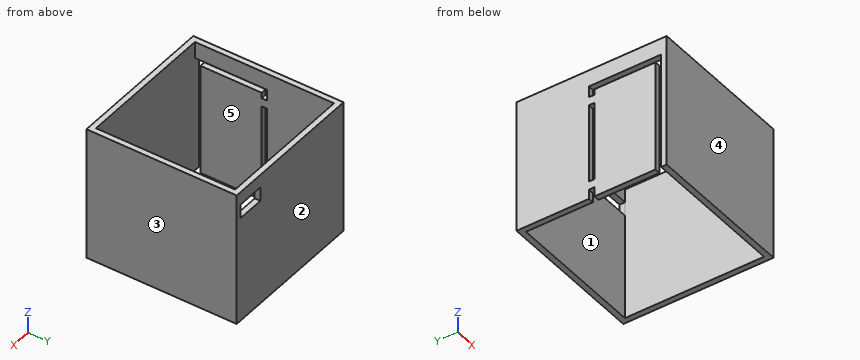
```python
from build123d import *

# Parameters (mm, degrees)
F0_W     = 50
F0_H     = 2
F1_DEPTH = 48
F3_W     = 2
F3_H     = 40
F3_H_2   = 3.4556204919
F3_H_3   = 28.4943341073
F3_H_4   = 2.0500454009
F4_DEPTH = 25
F5_W     = 10
F5_H     = 5
F6_DEPTH = 2


with BuildPart() as f1:
    # F0 (on Top) → F1 (new body)
    with BuildSketch(Plane.XY):
        with Locations((-0.1711930672, -2.4346486163)):
            Rectangle(F0_W, F0_H)
        Polygon((-27.1711930672, -3.4346486163), (-25.1711930672, -3.4346486163), (-25.1711930672, -1.4346486163), (-25.1711930672, 48.5653513837), (-25.1711930672, 50.5653513837), (-27.1711930672, 50.5653513837), align=None)
        Polygon((24.8288069328, -1.4346486163), (24.8288069328, -3.4346486163), (26.8288069328, -3.4346486163), (26.8288069328, 50.5653513837), (24.8288069328, 50.5653513837), (24.8288069328, 48.5653513837), align=None)
        with Locations((-0.1711930672, 49.5653513837)):
            Rectangle(F0_W, F0_H)
    extrude(amount=F1_DEPTH)

    # F3 (on face) → F4 (cut)
    with BuildSketch(Plane(origin=(-27.1711930672, 0, 0), x_dir=(0, -1, 0), z_dir=(-1, 0, 0))):
        with Locations((0.4346486163, 20)):
            Rectangle(F3_W, F3_H)
        with Locations((-23.5653513837, 1.7278102459)):
            Rectangle(F3_W, F3_H_2)
        with Locations((-23.5653513837, 20.7027875455)):
            Rectangle(F3_W, F3_H_3)
        with Locations((-23.5653513837, 38.9749772996)):
            Rectangle(F3_W, F3_H_4)
        Polygon((-0.5653513837, 40), (1.4346486163, 40), (1.4346486163, 42), (-24.5653513837, 42), (-24.5653513837, 40), (-22.5653513837, 40), align=None)
    extrude(amount=-F4_DEPTH, mode=Mode.SUBTRACT)

    # F5 (on face) → F6 (cut)
    with BuildSketch(Plane(origin=(0, 50.5653513837, 0), x_dir=(-1, 0, 0), z_dir=(0, 1, 0))):
        with Locations((-19.8940047994, 40.8047514008)):
            Rectangle(F5_W, F5_H)
    extrude(amount=-F6_DEPTH, mode=Mode.SUBTRACT)


solid = f1.part
```
Here's how the part is built. I have some questions about the finished solid (model axes, mm). Face numbers are marked on the shaded views. A direction names the side the tool comes from. Round coordinates to 2 decimals unless told otherwise and drop trailing zeros. Order: outer loops, then holes, each group sorted by start corner. A loop starts at its lowest first (then second) coordinate and runs counter-clockwise, first axis right, second up. Notation, with made-up numbers: (89, -30.75) -> (131, -30.75) arc R16 ccw to (131, -24.75) -> close; hole circle Ø10 at (3, 23.25). An arc over 180 degrees is marked (long way). Use a Markdown table: item, result. Add a question column.
(1) Suppose I cut it at C-C, the plane y = 4. Please give me the cut outline in (x, z), and give its area (3 significant figures).
(2) For the marked faces 4 and 5, which set-ups out of +Z, -Z, +X, -X, +Y, -Y let a thin tool reach every point of the face, with its end or its side?
(3) I need wall thicknesses on line 1 along Y through (x, z) = (-11, 38.5); line 2 along X through (y, z) = (34, 22); line 3 along X through (y, z) = (-1, 13). Which ranges of each line are inside material? Lowest first, please.
(4) Suppose I cut it at B-B, the plane x = 12. Please give me the cut outline in (y, z).
(5) Suppose I cut it at D-D, the plane y = 36. Please give me the cut outline in (x, z).
(6) If we mould it in two halves opening along X, with no side actions, what happens to the marked faces 1, 2 and 3? For each: released by +X, released by -X, zero draft, split by the parting line, or undercut.
(7) Suppose I cut it at A-A, the plane z = 21. Please give me the cut outline in (x, y).
Verdict:
| question | item | result |
|---|---|---|
| 1 | outline | (-27.17, 0) -> (-25.17, 0) -> (-25.17, 40) -> (-27.17, 40) -> close; (-27.17, 42) -> (-25.17, 42) -> (-25.17, 48) -> (-27.17, 48) -> close; (24.83, 0) -> (26.83, 0) -> (26.83, 48) -> (24.83, 48) -> close |
| 1 | area | 188 mm2 |
| 2 | face 4 | +Z, -Z, +X, -X, -Y |
| 2 | face 5 | +Z, -Z |
| 3 | line 1 | -3.43 to -1.43, 48.57 to 50.57 |
| 3 | line 2 | -27.17 to -25.17, 24.83 to 26.83 |
| 3 | line 3 | 24.83 to 26.83 |
| 4 | outline | (-3.43, 0) -> (-1.43, 0) -> (-1.43, 48) -> (-3.43, 48) -> close; (48.57, 0) -> (50.57, 0) -> (50.57, 48) -> (48.57, 48) -> close |
| 5 | outline | (-27.17, 0) -> (-25.17, 0) -> (-25.17, 48) -> (-27.17, 48) -> close; (24.83, 0) -> (26.83, 0) -> (26.83, 48) -> (24.83, 48) -> close |
| 6 | face 1 | undercut |
| 6 | face 2 | zero draft |
| 6 | face 3 | released by +X |
| 7 | outline | (-27.17, -3.43) -> (26.83, -3.43) -> (26.83, 50.57) -> (-27.17, 50.57) -> (-27.17, 24.57) -> (-25.17, 24.57) -> (-25.17, 48.57) -> (24.83, 48.57) -> (24.83, -1.43) -> (-27.17, -1.43) -> close; (-27.17, 0.57) -> (-25.17, 0.57) -> (-25.17, 22.57) -> (-27.17, 22.57) -> close |
